Verification items for the finished model (mm, model axes). A direction names the side the tool comes from. Round coordinates to 2 decimals unless told otherwise and drop trailing zeros. Loops run counter-clockwise (first coordinate to the right, second up) from the corner with the lowest first, then second, coordinate; pieces in that order, holes last. Notation, with made-up numbers: M 41.25,47.5 L 90.25,47.5 A11 ccw 90.25,60.5 Z; hole C -4,-6 d5. An arc over 180 degrees is marked long. Answer as CSV lines item,"result".
```python
from build123d import *

# Parameters (mm, degrees)
SKETCH1_R           = 35
SKETCH1_R_2         = 20
BOSS_EXTRUDE1_DEPTH = 75
BOSS_EXTRUDE2_DEPTH = 34
CUT_EXTRUDE1_REACH  = 120.808
SKETCH2_R           = 7.5
CUT_EXTRUDE2_REACH  = 142.947
SKETCH3_R           = 7.5


with BuildPart() as part:
    # Sketch1 → Boss-Extrude1 (new body)
    # profile 1 of 3: a face of its own
    with BuildSketch(Plane(origin=(0, 0, 0), x_dir=(1, 0, 0), z_dir=(0, 1, 0))):
        Circle(SKETCH1_R)
        with Locations(Location((0, 0, 0), (0, 0, 270))):
            Circle(SKETCH1_R_2, mode=Mode.SUBTRACT)
    # profile 2 of 3: a face of its own
    with BuildSketch(Plane(origin=(0, 0, 0), x_dir=(1, 0, 0), z_dir=(0, 1, 0))):
        with BuildLine():
            Line((-30.594117082, 17), (-55.668329577, 17))
            ThreePointArc((-55.668329577, 17), (-72.668329577, 0), (-55.668329577, -17))
            Line((-55.668329577, -17), (-55.547670544, -16.9995718))
            Line((-55.547670544, -16.9995718), (-30.643296936, -16.911190168))
            ThreePointArc((-30.643296936, -16.911190168), (-32.754908272, -12.333530885), (-34.186985828, -7.5))
            Line((-34.186985828, -7.5), (-55.668329577, -7.5))
            ThreePointArc((-55.668329577, -7.5), (-63.168329577, 0), (-55.668329577, 7.5))
            Line((-55.668329577, 7.5), (-34.186985828, 7.5))
            ThreePointArc((-34.186985828, 7.5), (-32.736987087, 12.381020816), (-30.594117082, 17))
        make_face()
    # profile 3 of 3: a face of its own
    with BuildSketch(Plane(origin=(0, 0, 0), x_dir=(1, 0, 0), z_dir=(0, 1, 0))):
        with BuildLine():
            ThreePointArc((-34.186985828, -7.5), (-35, 0), (-34.186985828, 7.5))
            Line((-34.186985828, 7.5), (-55.668329577, 7.5))
            ThreePointArc((-55.668329577, 7.5), (-50.365028718, 5.303300859), (-48.168329577, 0))
            ThreePointArc((-48.168329577, 0), (-50.365028718, -5.303300859), (-55.668329577, -7.5))
            Line((-55.668329577, -7.5), (-34.186985828, -7.5))
        make_face()
    extrude(amount=BOSS_EXTRUDE1_DEPTH)

    # Sketch1_4 → Boss-Extrude2 (add)
    with BuildSketch(Plane(origin=(0, 0, 0), x_dir=(1, 0, 0), z_dir=(0, 1, 0))):
        with BuildLine():
            ThreePointArc((-7.5, -34.186985828), (-15.446901808, -31.406897722), (-22.5, -26.809513237))
            Line((-22.5, -26.809513237), (-22.5, -72))
            Line((-22.5, -72), (-7.5, -72))
            Line((-7.5, -72), (-7.5, -34.186985828))
        make_face()
        with BuildLine():
            Line((22.5, -72), (22.5, -26.809513237))
            ThreePointArc((22.5, -26.809513237), (15.446901808, -31.406897722), (7.5, -34.186985828))
            Line((7.5, -34.186985828), (7.5, -72))
            Line((7.5, -72), (22.5, -72))
        make_face()
    extrude(amount=BOSS_EXTRUDE2_DEPTH)

    # Sketch2 → Cut-Extrude1 (cut, up to next)
    with BuildSketch(Plane.ZY.offset(22.5), mode=Mode.PRIVATE) as cut_extrude1_sk1:
        with BuildLine():
            Line((72, 0), (72, 17))
            ThreePointArc((72, 17), (67.02081528, 4.97918472), (55, 0))
            Line((55, 0), (72, 0))
        make_face()
    cut_extrude1_tool1 = extrude(cut_extrude1_sk1.sketch, amount=-CUT_EXTRUDE1_REACH, mode=Mode.PRIVATE) & part.part
    # Sketch2 → Cut-Extrude1 (cut, up to next)
    with BuildSketch(Plane.ZY.offset(22.5), mode=Mode.PRIVATE) as cut_extrude1_sk2:
        with BuildLine():
            Line((72, 34), (55, 34))
            ThreePointArc((55, 34), (67.02081528, 29.02081528), (72, 17))
            Line((72, 17), (72, 34))
        make_face()
    cut_extrude1_tool2 = extrude(cut_extrude1_sk2.sketch, amount=-CUT_EXTRUDE1_REACH, mode=Mode.PRIVATE) & part.part
    # Sketch2 → Cut-Extrude1 (cut, up to next)
    with BuildSketch(Plane.ZY.offset(22.5), mode=Mode.PRIVATE) as cut_extrude1_sk3:
        with Locations((55, 17)):
            Circle(SKETCH2_R)
    cut_extrude1_tool3 = extrude(cut_extrude1_sk3.sketch, amount=-CUT_EXTRUDE1_REACH, mode=Mode.PRIVATE) & part.part
    add(cut_extrude1_tool1.solids().sort_by_distance((-22.5, 3.797255, 68.202745))[0], mode=Mode.SUBTRACT)
    add(cut_extrude1_tool2.solids().sort_by_distance((-22.5, 30.202745, 68.202745))[0], mode=Mode.SUBTRACT)
    add(cut_extrude1_tool3.solids().sort_by_distance((-22.5, 17, 55))[0], mode=Mode.SUBTRACT)

    # Sketch3 → Cut-Extrude2 (cut, up to next)
    with BuildSketch(Plane(origin=(22.5, 0, 0), x_dir=(0, 0, -1), z_dir=(1, 0, 0)), mode=Mode.PRIVATE) as cut_extrude2_sk1:
        with Locations(Location((-55, 17, 0), (0, 0, 180))):
            Circle(SKETCH3_R)
    cut_extrude2_tool1 = extrude(cut_extrude2_sk1.sketch, amount=-CUT_EXTRUDE2_REACH, mode=Mode.PRIVATE) & part.part
    # Sketch3 → Cut-Extrude2 (cut, up to next)
    with BuildSketch(Plane(origin=(22.5, 0, 0), x_dir=(0, 0, -1), z_dir=(1, 0, 0)), mode=Mode.PRIVATE) as cut_extrude2_sk2:
        with BuildLine():
            ThreePointArc((-72, 17), (-67.02081528, 29.02081528), (-55, 34))
            Line((-55, 34), (-72, 34))
            Line((-72, 34), (-72, 17))
        make_face()
    cut_extrude2_tool2 = extrude(cut_extrude2_sk2.sketch, amount=-CUT_EXTRUDE2_REACH, mode=Mode.PRIVATE) & part.part
    # Sketch3 → Cut-Extrude2 (cut, up to next)
    with BuildSketch(Plane(origin=(22.5, 0, 0), x_dir=(0, 0, -1), z_dir=(1, 0, 0)), mode=Mode.PRIVATE) as cut_extrude2_sk3:
        with BuildLine():
            ThreePointArc((-55, 0), (-67.02081528, 4.97918472), (-72, 17))
            Line((-72, 17), (-72, 0))
            Line((-72, 0), (-55, 0))
        make_face()
    cut_extrude2_tool3 = extrude(cut_extrude2_sk3.sketch, amount=-CUT_EXTRUDE2_REACH, mode=Mode.PRIVATE) & part.part
    add(cut_extrude2_tool1.solids().sort_by_distance((22.5, 17, 55))[0], mode=Mode.SUBTRACT)
    add(cut_extrude2_tool2.solids().sort_by_distance((22.5, 30.202745, 68.202745))[0], mode=Mode.SUBTRACT)
    add(cut_extrude2_tool3.solids().sort_by_distance((22.5, 3.797255, 68.202745))[0], mode=Mode.SUBTRACT)


solid = part.part
```
1) Go/stop test with flat-tipped pins: pin 1 (8 mm diameter, centred on y = 36, z = 50.5, fed in from +X); pin 2 (5 mm diameter, centred on x = 23.5, y = 25, fed in from -Z); pin 3 (12 mm diameter, centred on x = -12, z = 42, fed in from +Y). Record where each tip stops, or that it passes through.
Here are the results:
pin 1,"stops at x = 22.5"
pin 2,"stops at z = -28"
pin 3,"stops at y = 34"
2) Section check D-D (z = 2). Record the cut outline in (x, y).
Here are the results:
outline,"M -72.55,0 L -62.9,0 L -62.9,75 L -72.55,75 Z; M -48.44,0 L -19.9,0 L -19.9,75 L -48.44,75 Z; M 19.9,0 L 34.94,0 L 34.94,75 L 19.9,75 Z"
3) Section check C-C (x = 0). Record the cut outline in (y, z).
Here are the results:
outline,"M 0,-35 L 75,-35 L 75,-20 L 0,-20 Z; M 0,20 L 75,20 L 75,35 L 0,35 Z"
4) Draft check along Z on faces 1 (the cylindrical face through (-72.664, 36.975, -0.374)), 2 (the flat face through (-15, 34, 44)), 3 (the cylindrical face through (15.105, 10.676, 59.032)), 4 (the cylindrical face through (-15.105, 24.436, 54.024)). Enter one of: +Z half, -Z half, draft (parallel to the pull), parting line (faces both ways), or undercut.
Here are the results:
face 1,"parting line"
face 2,"draft"
face 3,"undercut"
face 4,"undercut"
5) Material ranges on probe 1 along X at (y, z) = (21, 0); probe 2 along Z at (x, y) = (-0.5, 7); probe 3 along X at (y, z) = (63.5, 4), recorded low to high.
Here are the results:
probe 1,"x = -72.67 to -63.17, -48.17 to -20, 20 to 35"
probe 2,"z = -35 to -19.99, 19.99 to 35"
probe 3,"x = -72.19 to -62.01, -49.32 to -19.6, 19.6 to 34.77"
6) Section check B-B (x = 12.5). Record the cut outline in (y, z), plus the area to 3 significant figures.
Here are the results:
outline,"M 0,-32.69 L 75,-32.69 L 75,-15.61 L 0,-15.61 Z; M 0,15.61 L 75,15.61 L 75,32.69 L 34,32.69 L 34,55 A17 ccw 0,55 Z; hole C 17,55 d15"
area,"3,600 mm^2"
7) Set-up check for faces 5 (the flat face through (-7.5, 17, 45)), 6 (the cylindrical face through (29.886, 36.975, -18.216)), 7 (the flat face through (-22.5, 17, 44)): record each of +Z, -Z, +X, -X, +Y, -Y from which the full face is reachable in a straight line by a thin tool's end or side.
Here are the results:
face 5,"+Z, +Y, -Y"
face 6,"+Y"
face 7,"+Z, -X, +Y, -Y"
8) Section check A-A (y = 20.5). Record the cut outline in (x, z), plus the area to 3 significant figures.
Here are the results:
outline,"M -55.67,-17 L -30.59,-17 A35 ccw long 22.5,26.81 L 22.5,48.37 L 7.5,48.37 L 7.5,34.19 A35 ccw -7.5,34.19 L -7.5,48.37 L -22.5,48.37 L -22.5,26.81 A35 ccw -30.64,16.91 L -55.67,17 A17 ccw Z; M -22.5,61.63 L -7.5,61.63 L -7.5,71.64 L -22.5,71.64 Z; M 7.5,61.63 L 22.5,61.63 L 22.5,71.64 L 7.5,71.64 Z; hole C -55.67,0 d15; hole C 0,0 d40"
area,"4,430 mm^2"
